Verification items for the finished model (mm, model axes). Face numbers are marked on the shaded views. Coordinates: 2 decimals unless noted, no trailing zeros. Order: outer loops, then holes, each group sorted by start corner. A loop starts at its lowest first (then second) coordinate and runs counter-clockwise, first axis right, second up. Notation, with made-up numbers: (38.5, -13) - (63.5, -13) arc R15 cw to (63.5, -5) - close; hole circle Ø11 at (58.5, 35.5). An arc over 180 degrees is marked (long way). Answer as CSV lines item,"result". Start each with the question number.
1. Mould release check, pull along X, two halves, no side actions. Record for the marked faces 1, 2 and 3: pulls with the +X half, pulls with the -X half, needs draft (parallel to the pull), parting line crosses it, or undercut.
2. Material ranges on L1, parallel to Y at x = 300, z = -8; L2, parallel to X at y = 40.5, z = -10; L3, parallel to X at y = 27, z = 2, recorded low to high. Write a range as [from, to].
3. Section check B-B (z = -17). Count the separate pieces of the cut face and the enclosed holes in it, and give its area (3 significant figures).
4. Section check C-C (x = 202.5). Record the cut outline in (y, z).
5. Go/stop test with flat-tipped pins: pin 1 (4 mm diameter, centred on x = 68.5, z = -27.5, fed in from +Y); pin 2 (3 mm diameter, centred on x = 273.5, y = 4, fed in from +Z); pin 3 (1 mm diameter, centred on x = 73.5, y = -23, fed in from -Z); pin 4 (6 mm diameter, centred on x = 300, y = 0, fed in from -Z). Record where each tip stops, or that it passes through.
6. Section check A-A (x = 300). Record the cut outline in (y, z).
from build123d import *

# Parameters (mm, degrees)
SKETCH_2_R          = 5
EXTRUDE_1_DEPTH     = 200
SKETCH_3_R          = 10
EXTRUDE_2_DEPTH     = 20
SKETCH_4_R          = 5
CUT_EXTRUDE_1_DEPTH = 40


with BuildPart() as part:
    # Эскиз1 → Повернуть1 (revolve)
    with BuildSketch(Plane.XY, mode=Mode.PRIVATE) as revolve_1_sk:
        Polygon((0, 40), (5, 45), (20, 45), (20, 40), (23, 40), (23, 45), (35, 45), (35, 40), (38, 40), (38, 45), (50, 45), (50, 40), (53, 40), (53, 45), (65, 45), (65, 40), (68, 40), (68, 45), (80, 45), (80, 40), (83, 40), (83, 45), (95, 45), (100, 40), (100, 0), (0, 0), align=None)
    revolve(revolve_1_sk.sketch.rotate(Axis((-82.862068966, 0, 0), (1, 0, 0)), 90), axis=Axis((-82.862068966, 0, 0), (1, 0, 0)))

    # Эскиз2 → Бобышка-Вытянуть1 (add)
    with BuildSketch(Plane(origin=(100, 0, 0), x_dir=(0, 0, -1), z_dir=(1, 0, 0))):
        with Locations(Location((0, 0, 0), (0, 0, 180))):
            Circle(SKETCH_2_R)
    extrude(amount=EXTRUDE_1_DEPTH)

    # Эскиз3 → Бобышка-Вытянуть2 (add, symmetric)
    with BuildSketch(Plane.XY):
        with Locations((300, 0)):
            Circle(SKETCH_3_R)
    extrude(amount=EXTRUDE_2_DEPTH, both=True)

    # Эскиз4 → Вырез-Вытянуть1 (cut)
    with BuildSketch(Plane.XY.offset(20)):
        with Locations((300, 0)):
            Circle(SKETCH_4_R)
    extrude(amount=-CUT_EXTRUDE_1_DEPTH, mode=Mode.SUBTRACT)


solid = part.part
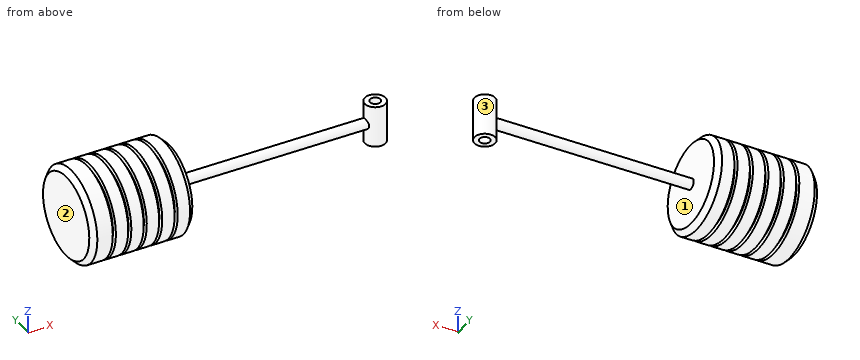
Evaluation:
1,face 1,"undercut"
1,face 2,"pulls with the -X half"
1,face 3,"undercut"
2,L1,"y = [-10, -5], [5, 10]"
2,L2,"x = [1.72, 20], [23, 35], [38, 50], [53, 65], [68, 80], [83, 98.28]"
2,L3,"x = [0, 100]"
3,separate pieces,"2"
3,enclosed holes,"1"
3,area,"8,350 mm²"
4,outline,"circle Ø10 at (0, 0)"
5,pin 1,"stops at y = 37.08"
5,pin 2,"stops at z = 4.33"
5,pin 3,"stops at z = -38.97"
5,pin 4,"passes through"
6,outline,"(-10, -20) - (-5, -20) - (-5, 20) - (-10, 20) - close; (5, -20) - (10, -20) - (10, 20) - (5, 20) - close"
